CAD build for the part. Positions are in the model's coordinates, mm. Face numbers are marked on the shaded views. Give positions to 0.01 mm unless a question says otherwise; leave off trailing zeros. Write each loop counter-clockwise with the first axis right and the second up, starting at its lowest first coordinate (ties: lowest second). Pieces come first, ordered by that corner, then holes. Notation, with made-up numbers: (74.5, 25) -> (109.5, 25) arc R21 ccw to (109.5, 50) -> close; hole circle Ø4 at (15.25, -18.5). An arc over 180 degrees is marked (long way). Answer as a JSON object with one key per item and string values.
Autodesk Inventor part; units mm, degrees
ref_plane "YZ Plane" through (0, 0, 0) normal (1, 0, 0) x (0, 1, 0)
ref_plane "XZ Plane" through (0, 0, 0) normal (0, 1, 0) x (-1, 0, 0)
ref_plane "XY Plane" through (0, 0, 0) normal (0, 0, 1) x (1, 0, 0)
ref_plane "Work Plane1" through (0, 0, 0) normal (0, 0, 1) x (1, 0, 0)
sketch "Sketch1" plane through (0, 0, 0) normal (0, 0, 1) x (1, 0, 0)
  line L0 (22.8064, -35.5) -> (-89.6938, -35.5)
  line L1 (-89.6938, -35.5) -> (-89.6938, 0)
  line L2 (-89.6938, 0) -> (-74.2938, 0)
  line L3 (22.8064, 0) -> (22.8064, -35.5)
  circle A0 centre (11.5562, -18) radius 2 construction
  line L4 (-53.1938, -16) -> (-53.1938, -30) construction
  arc A1 (-56.1938, -30) -> (-53.1938, -30) centre (-54.6938, -30) ccw construction
  line L5 (-56.1938, -30) -> (-56.1938, -16) construction
  arc A2 (-53.1938, -16) -> (-56.1938, -16) centre (-54.6938, -16) ccw construction
  line L6 (7.0562, -16) -> (7.0562, -30) construction
  arc A3 (4.0562, -30) -> (7.0562, -30) centre (5.5562, -30) ccw construction
  line L7 (4.0562, -30) -> (4.0562, -16) construction
  arc A4 (7.0562, -16) -> (4.0562, -16) centre (5.5562, -16) ccw construction
  line L8 (-13.1938, -16) -> (-13.1938, -30) construction
  arc A5 (-16.1938, -30) -> (-13.1938, -30) centre (-14.6938, -30) ccw construction
  line L9 (-16.1938, -30) -> (-16.1938, -16) construction
  arc A6 (-13.1938, -16) -> (-16.1938, -16) centre (-14.6938, -16) ccw construction
  arc A7 (19.0562, -16) -> (16.0562, -16) centre (17.5562, -16) ccw construction
  line L10 (19.0562, -16) -> (19.0562, -30) construction
  arc A8 (16.0562, -30) -> (19.0562, -30) centre (17.5562, -30) ccw construction
  line L11 (16.0562, -30) -> (16.0562, -16) construction
  line L12 (22.8064, -40) -> (22.8064, 45) construction
  line L13 (22.8064, 45) -> (-120, 45) construction
  line L14 (-120, 27.5563) -> (-120, 45) construction
  line L15 (-120, 27.5563) -> (-95.2035, 27.5563) construction
  arc A9 (-85.0841, 27.5563) -> (-95.2035, 27.5563) centre (-90.1438, 25.4) ccw construction
  line L16 (-85.0841, 27.5563) -> (17.8062, 27.5563) construction
  line L17 (17.8062, 27.5563) -> (17.8062, -11) construction
  line L18 (17.8062, -11) -> (-120, -11) construction
  line L19 (-120, -40) -> (-120, -11) construction
  line L20 (22.8064, -40) -> (-120, -40) construction
  circle A10 centre (-111.1938, -18) radius 2 construction
  circle A11 centre (-98.1938, -18) radius 2 construction
  circle A12 centre (-61.1938, -18) radius 2 construction
  circle A13 centre (-48.1938, -18) radius 2 construction
  circle A14 centre (-21.1938, -18) radius 2 construction
  circle A15 centre (-8.1938, -18) radius 2 construction
  circle A16 centre (-21.1938, 33.6563) radius 2 construction
  circle A17 centre (-8.1938, 33.6563) radius 2 construction
  circle A18 centre (-61.1938, 33.6563) radius 2 construction
  circle A19 centre (-48.1938, 33.6563) radius 2 construction
  circle A20 centre (-111.1938, 33.6563) radius 2 construction
  circle A21 centre (-98.1938, 33.6563) radius 2 construction
  circle A22 centre (-90.1438, -25.4) radius 5.5 construction
  line L21 (-84.6938, 26.6563) -> (-89.6938, 26.6563) construction
  line L22 (-89.6938, 26.6563) -> (-89.6938, -11) construction
  line L23 (-84.6938, -11) -> (-89.6938, -11) construction
  line L24 (-84.6938, 26.6563) -> (-84.6938, -11) construction
  line L25 (-84.6938, 26.6563) -> (-84.6938, -11) construction
  circle A23 centre (1.3062, 0) radius 6 construction
  circle A24 centre (-68.1938, 0) radius 6 construction
  arc A25 (-4.7938, 0) -> (7.4062, 0) centre (1.3062, 0) ccw
  arc A26 (-74.2938, 0) -> (-62.0938, 0) centre (-68.1938, 0) ccw
  line L26 (-148.5613, 0) -> (51.3677, 0) construction
  line L27 (7.4062, 0) -> (22.8064, 0)
  line L28 (-62.0938, 0) -> (-4.7938, 0)
  point P0 (0, 0)
  point P1 (17.5562, -31.5)
  dimension "d0" = 0
  dimension "d1" = 0
  dimension "d2" = 4
  dimension "d3" = 0.1
  dimension "d4" = 0.1
extrude "Main Body" add sketch "Sketch1" along normal blind 5
sketch "Sketch2" plane through (0, 0, 0) normal (0, 0, -1) x (-1, 0, 0)
  line L0 (56.1938, -30) -> (56.1938, -16) construction
  arc A0 (53.1938, -30) -> (56.1938, -30) centre (54.6938, -30) ccw construction
  line L1 (53.1938, -16) -> (53.1938, -30) construction
  arc A1 (56.1938, -16) -> (53.1938, -16) centre (54.6938, -16) ccw construction
  arc A2 (13.1938, -30) -> (16.1938, -30) centre (14.6938, -30) ccw construction
  line L2 (13.1938, -16) -> (13.1938, -30) construction
  arc A3 (16.1938, -16) -> (13.1938, -16) centre (14.6938, -16) ccw construction
  line L3 (16.1938, -30) -> (16.1938, -16) construction
  line L4 (14.6938, -16) -> (14.6938, -30) construction
  line L5 (54.6938, -16) -> (54.6938, -30) construction
  line L6 (14.6938, -29) -> (14.6938, -17) construction
  line L7 (13.2438, -29) -> (13.2438, -17)
  line L8 (16.1438, -17) -> (16.1438, -29)
  arc A4 (13.2438, -29) -> (16.1438, -29) centre (14.6938, -29) ccw
  arc A5 (16.1438, -17) -> (13.2438, -17) centre (14.6938, -17) ccw
  line L9 (54.6938, -29) -> (54.6938, -17) construction
  line L10 (53.2438, -29) -> (53.2438, -17)
  line L11 (56.1438, -17) -> (56.1438, -29)
  arc A6 (53.2438, -29) -> (56.1438, -29) centre (54.6938, -29) ccw
  arc A7 (56.1438, -17) -> (53.2438, -17) centre (54.6938, -17) ccw
  line L12 (14.6938, -17) -> (54.6938, -17) construction
  point P0 (0, 0)
  point P1 (14.6938, -23)
  point P2 (54.6938, -23)
  dimension "d7" = 0.05
  dimension "d8" = 0.05
  dimension "d9" = 1
extrude "Alignment Tabs" add sketch "Sketch2" along normal blind 1.8
sketch "Sketch3" plane through (0, 0, 5) normal (0, 0, -1) x (-1, 0, 0)
  circle A0 centre (61.1938, -18) radius 2 construction
  circle A1 centre (8.1938, -18) radius 2 construction
  line L0 (61.1938, -16.5) -> (61.1938, -19.5) construction
  line L1 (59.4438, -16.5) -> (59.4438, -19.5)
  line L2 (62.9438, -19.5) -> (62.9438, -16.5)
  arc A2 (62.9438, -16.5) -> (59.4438, -16.5) centre (61.1938, -16.5) ccw
  arc A3 (59.4438, -19.5) -> (62.9438, -19.5) centre (61.1938, -19.5) ccw
  line L3 (8.1938, -16.5) -> (8.1938, -19.5) construction
  line L4 (6.4438, -16.5) -> (6.4438, -19.5)
  line L5 (9.9438, -19.5) -> (9.9438, -16.5)
  arc A4 (9.9438, -16.5) -> (6.4438, -16.5) centre (8.1938, -16.5) ccw
  arc A5 (6.4438, -19.5) -> (9.9438, -19.5) centre (8.1938, -19.5) ccw
  point P0 (0, 0)
  dimension "d12" = 3.5
  dimension "d13" = 3.5
  dimension "d14" = 3
  dimension "d15" = 3
extrude "Slots for Screws M3" cut sketch "Sketch3" along normal through all
equation "\"d4\" = d3"
equation "\"d8\" = d7"
equation "\"d13\" = d12"
equation "\"d15\" = d14"
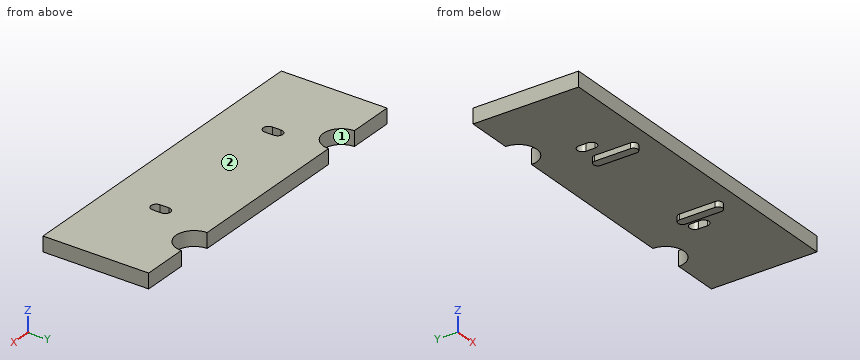
1) Slice it at B-B (y = -2.5). List the corners of the cut face in (x, z).
Model answer:
{"outline": "(-89.69, 0) -> (-73.76, 0) -> (-73.76, 5) -> (-89.69, 5) -> close; (-62.63, 0) -> (-4.26, 0) -> (-4.26, 5) -> (-62.63, 5) -> close; (6.87, 0) -> (22.81, 0) -> (22.81, 5) -> (6.87, 5) -> close"}
2) Slice it at A-A (z = 1.75). List the corners of the cut face in (x, y), then the cut area to 3 significant figures.
Model answer:
{"outline": "(-89.69, -35.5) -> (22.81, -35.5) -> (22.81, 0) -> (7.41, 0) arc R6.1 cw to (-4.79, 0) -> (-62.09, 0) arc R6.1 cw to (-74.29, 0) -> (-89.69, 0) -> close; hole (-62.94, -19.5) arc R1.75 ccw to (-59.44, -19.5) -> (-59.44, -16.5) arc R1.75 ccw to (-62.94, -16.5) -> close; hole (-9.94, -19.5) arc R1.75 ccw to (-6.44, -19.5) -> (-6.44, -16.5) arc R1.75 ccw to (-9.94, -16.5) -> close", "area": "3,840 mm2"}
3) Slice it at D-D (x = -51.5). List the corners of the cut face in (y, z).
Model answer:
{"outline": "(-35.5, 0) -> (0, 0) -> (0, 5) -> (-35.5, 5) -> close"}
4) Pin check, flat tips, straight feed: pin 1 (1.4 mm diameter, centred on y = -24.5, z = -1, fed in from +X); pin 2 (1.4 mm diameter, centred on y = -22.5, z = -1, fed in from -X). Stop position of each tip, or through.
Model answer:
{"pin 1": "stops at x = -13.24", "pin 2": "stops at x = -56.14"}
5) Wall check: probe 1 along X at (y, z) = (-23, -1.25); probe 2 along Z at (x, y) = (-36.5, -23); probe 3 along Y at (x, z) = (-63, 1.75). Give the ranges that are in metal, low to high.
Model answer:
{"probe 1": "x = -56.14 to -53.24, -16.14 to -13.24", "probe 2": "z = 0 to 5", "probe 3": "y = -35.5 to -3.2"}
6) Slice it at C-C (y = -8). List the corners of the cut face in (x, z), then the cut area to 4 significant figures.
Model answer:
{"outline": "(-89.69, 0) -> (22.81, 0) -> (22.81, 5) -> (-89.69, 5) -> close", "area": "562.5 mm2"}
7) Mould opens along X. For the marked faces 1 and 2 say: released by +X, released by -X, zero draft, split by the parting line, or undercut.
Model answer:
{"face 1": "undercut", "face 2": "zero draft"}
